from build123d import *

# Parameters (mm, degrees)
BOSS_EXTRUDE1_DEPTH                             = 0.8
BOSS_EXTRUDE1_2_DEPTH                           = 0.8
BOSS_EXTRUDE3_DEPTH                             = 1
BOSS_EXTRUDE3_DEPTH_BACK                        = 0.2
FILLET1_R                                       = 2
CUT_EXTRUDE1_DEPTH                              = 0.2
BOSS_EXTRUDE4_DEPTH                             = 0.75
CSK_FOR_M2_FLAT_HEAD_MACHINE_SCREW1_D           = 2.4
CSK_FOR_M2_FLAT_HEAD_MACHINE_SCREW1_DEPTH       = 4
CSK_FOR_M2_FLAT_HEAD_MACHINE_SCREW1_CSINK_D     = 4.4
CSK_FOR_M2_FLAT_HEAD_MACHINE_SCREW1_CSINK_ANGLE = 90
CSK_FOR_M2_FLAT_HEAD_MACHINE_SCREW1_TIP         = 0.721032743


with BuildPart() as part:
    # Sketch1 → Boss-Extrude1 (new body)
    with BuildSketch(Plane.XY):
        with BuildLine():
            Line((11.255059848, 53.733600539), (13.255059848, 53.733600539))
            Line((13.255059848, 53.733600539), (13.255059848, 50.733600539))
            Line((13.255059848, 50.733600539), (11.255059848, 50.733600539))
            ThreePointArc((11.255059848, 50.733600539), (9.755059848, 52.233600539), (11.255059848, 53.733600539))
        make_face()
    extrude(amount=-BOSS_EXTRUDE1_DEPTH)



with BuildPart() as body_2:
    # Sketch1 → Boss-Extrude1 2 (new body)
    with BuildSketch(Plane.XY):
        with BuildLine():
            Line((11.255059848, 47.733600539), (13.255059848, 47.733600539))
            Line((13.255059848, 47.733600539), (13.255059848, 44.733600539))
            Line((13.255059848, 44.733600539), (11.255059848, 44.733600539))
            ThreePointArc((11.255059848, 44.733600539), (9.755059848, 46.233600539), (11.255059848, 47.733600539))
        make_face()
    extrude(amount=-BOSS_EXTRUDE1_2_DEPTH)


with BuildPart() as part_1:
    add(part.part)

    add(body_2.part)  # Boss-Extrude3 merges body 2
    # Sketch2 → Boss-Extrude3 (add, two sides)
    with BuildSketch(Plane.XY) as boss_extrude3_sk:
        Polygon((-5.444940152, 19.108600539), (13.255059848, 19.108600539), (13.255059848, 57.908600539), (10.255059848, 57.908600539), (-5.444940152, 40.168487545), align=None)
    extrude(amount=BOSS_EXTRUDE3_DEPTH)
    extrude(boss_extrude3_sk.sketch, amount=-BOSS_EXTRUDE3_DEPTH_BACK)

    # Fillet1
    fillet1_edges = [part_1.edges().sort_by_distance(p)[0] for p in [
        (-5.444940152, 19.108600539, 0.4),
        (13.255059848, 19.108600539, 0.4),
    ]]
    fillet(fillet1_edges, radius=FILLET1_R)

    # Sketch3 → Cut-Extrude1 (cut)
    with BuildSketch(Plane(origin=(0, 0, 0), x_dir=(-1, 0, 0), z_dir=(0, 0, -1))):
        Polygon((-13.255059848, 33.233600539), (-13.255059848, 19.108600539), (5.444940152, 19.108600539), (3.444940152, 20.619295727), align=None)
    extrude(amount=CUT_EXTRUDE1_DEPTH, mode=Mode.SUBTRACT)

    # Sketch4 → Boss-Extrude4 (add)
    with BuildSketch(Plane.XY.offset(1)):
        with BuildLine():
            Line((-6.444940152, 39.038544042), (-6.444940152, 21.108600539))
            ThreePointArc((-6.444940152, 21.108600539), (-6.247457228, 20.03813427), (-5.681008129, 19.108600539))
            Line((-5.681008129, 19.108600539), (13.491127826, 19.108600539))
            ThreePointArc((13.491127826, 19.108600539), (14.057576925, 20.03813427), (14.255059848, 21.108600539))
            Line((14.255059848, 21.108600539), (14.255059848, 57.908600539))
            Line((14.255059848, 57.908600539), (10.255059848, 57.908600539))
            Line((10.255059848, 57.908600539), (-6.444940152, 39.038544042))
        make_face()
    extrude(amount=-BOSS_EXTRUDE4_DEPTH)

    # CSK for M2 Flat Head Machine Screw1
    with Locations(Plane(origin=(-1.094940152, -30.37062024, 1), x_dir=(1, 0, 0), z_dir=(0, 0, 1))):
        with Locations((11.85, 56.367589763), (6.85, 52.590851795)):
            CounterSinkHole(CSK_FOR_M2_FLAT_HEAD_MACHINE_SCREW1_D / 2, CSK_FOR_M2_FLAT_HEAD_MACHINE_SCREW1_CSINK_D / 2, depth=CSK_FOR_M2_FLAT_HEAD_MACHINE_SCREW1_DEPTH, counter_sink_angle=CSK_FOR_M2_FLAT_HEAD_MACHINE_SCREW1_CSINK_ANGLE)
            with Locations((0, 0, -(CSK_FOR_M2_FLAT_HEAD_MACHINE_SCREW1_DEPTH + CSK_FOR_M2_FLAT_HEAD_MACHINE_SCREW1_TIP / 2))):  # 118° drill point
                Cone(0, CSK_FOR_M2_FLAT_HEAD_MACHINE_SCREW1_D / 2, CSK_FOR_M2_FLAT_HEAD_MACHINE_SCREW1_TIP, mode=Mode.SUBTRACT)


solid = part_1.part
Can you work these out from the model? Positions are in its coordinate system, mm. A direction names the side the tool comes from. Coordinates: 2 decimals unless noted, no trailing zeros. Order: outer loops, then holes, each group sorted by start corner. A loop starts at its lowest first (then second) coordinate and runs counter-clockwise, first axis right, second up. Notation, with made-up numbers: (-35, 23.25) -> (-1, 23.25) arc R6 ccw to (-1, 28.25) -> close; hole circle Ø4 at (-31.75, 48). An arc over 180 degrees is marked (long way). Use one line per item in the form item = value.
Q1. We'd pull the mould along Y, two halves only. Please class faces 6 (the face through (12, 57.909, 0)), 7 (the face through (9.755, 46.201, -0.496)), 8 (the face through (12, 46, -0.8)), 9 (the face through (9.755, 52.201, -0.496)): released by +Y, released by -Y, zero draft, split by the parting line, or undercut.
From the geometry:
face_6 = released by +Y
face_7 = undercut
face_8 = zero draft
face_9 = undercut
Q2. I need wall thicknesses on L1, parallel to Z at x = -1, y = 31.5; L2, parallel to Z at x = 6, y = 26; L3, parallel to Y at x = 10.5, z = 0.7. Which ranges of each line are inside material? Lowest first, please.
From the geometry:
L1 = -0.2 to 1
L2 = 0 to 1
L3 = 19.11 to 24.11, 27.88 to 57.91
Q3. Will these pins go through, and if not, where does the flat tip stop? P1, Ø0.9, axis at x = 12.5, y = 33, coming from the -Z side; P2, Ø4, axis at x = 6, y = 25, coming from the -Z side; P3, Ø0.5, axis at x = 12.5, z = -0.5, coming from the -Y side.
From the geometry:
P1 = -0.2
P2 = 0
P3 = 44.73
Q4. Imagine slicing it at C-C, the plane y = 50. List the corners of the cut face in (x, z) for me.
From the geometry:
outline = (3.26, -0.2) -> (13.26, -0.2) -> (13.26, 0.25) -> (14.26, 0.25) -> (14.26, 1) -> (3.26, 1) -> close
Q5. Imagine slicing it at B-B, the plane x = 2.25. List the corners of the cut face in (y, z) for me.
From the geometry:
outline = (19.11, 0) -> (24.92, 0) -> (24.92, -0.2) -> (48.86, -0.2) -> (48.86, 1) -> (19.11, 1) -> close
Q6. Which directions (+Z, -Z, +X, -X, +Y, -Y) give clear straight access to the entire face, cutting with the end or side of a thin tool? Please do faces 1 (the face through (4, 34, 1)), 2 (the face through (13.255, 43, 0)), 3 (the face through (6, 25, 0)), 4 (the face through (-5.07, 19.94, 0.07)), 5 (the face through (3.8, 19.109, 0.5)).
From the geometry:
face_1 = +Z, +X, -X, +Y, -Y
face_2 = -Z, +X, +Y, -Y
face_3 = -Z, +X, -Y
face_4 = -Z, -X, -Y
face_5 = +Z, -Z, +X, -X, -Y
Q7. Imagine slicing it at A-A, the plane y = 30.5. List the corners of the cut face in (x, z) for me, then the cut area to 3 significant figures.
From the geometry:
outline = (-6.44, 0.25) -> (-5.44, 0.25) -> (-5.44, -0.2) -> (9.64, -0.2) -> (9.64, 0) -> (13.26, 0) -> (13.26, 0.25) -> (14.26, 0.25) -> (14.26, 1) -> (-6.44, 1) -> close
area = 23.2 mm²
